from build123d import *

# Parameters (mm, degrees)
F1_DEPTH = 10
F2_T     = -1
F3_R     = 10.6640979673
F4_DEPTH = 25


with BuildPart() as f1:
    # F0 (on Top) → F1 (new body)
    with BuildSketch(Plane.XY):
        Polygon((-31.0254581273, 32.8216664493), (-59.7648322582, 20.7380689681), (-49.9673187733, 12.5734750181), (-42.7824743092, 8.6544696242), (-40.7788045704, 6.7279691546), (-40.7788045704, 2.8554322198), (-41.5555574, -1.3681541895), (-41.5555574, -3.4556735773), (-38.4888425469, -7.9726679251), (-31.0126114637, -14.5143707892), (-28.6823585629, -19.8181271553), (-26.0819279657, -26.5176091343), (-25.6298921539, -27.6821877156), (-16.0601455718, -22.7309465408), (-4.7972491011, -17.4878742546), (0, -16.4924804121), (12.7747104677, -16.4924804121), (15.1070067659, -18.5332398809), (16.0779468715, -21.3716309518), (16.0779468715, -23.5076975077), (15.1070067659, -26.5176091343), (18.6152737588, -32.1685001254), (18.6152737588, -43.598935008), (23.5140342265, -51.1103607714), (25.8403085172, -50.369720906), (28.2073356211, -49.6192015707), (31.2671549618, -48.984143883), (32.1908704937, -47.136709094), (32.7681936324, -45.3470014036), (34.5001667738, -44.6542128921), (35.8280129731, -42.9799742997), (36.2321399152, -40.0933548808), (35.2506898344, -37.0335392654), (33.0568552017, -33.1654660404), (30.863026157, -30.2788466215), (28.0862059444, -27.9229115695), (27.8792269528, -24.5023760945), (27.8792269528, -21.8466855586), (26.8400404602, -20.3456450254), (23.7224902958, -18.7291372567), (22.8264033794, -14.0075832605), (22.8264033794, 0), (33.3115458488, 5.0620483235), (45.0685583055, 10.6139723212), (46.1755990982, 11.7365671322), (45.0685583055, 13.5532263666), (27.7596209198, 22.3709885031), (6.5316753462, 32.8216664493), (-10.4506798089, 40.6596809626), align=None)
    extrude(amount=F1_DEPTH)

    # F2
    f2_openings = [f1.faces().sort_by_distance(p)[0] for p in [
        (-4.783125, 4.353197, 10),
    ]]
    offset(amount=F2_T, openings=f2_openings, kind=Kind.INTERSECTION)

    # F3 (on face) → F4 (cut)
    with BuildSketch(Plane.XY.offset(1)):
        with Locations((-9.2489561066, 8.1327119842)):
            Circle(F3_R)
    extrude(amount=-F4_DEPTH, mode=Mode.SUBTRACT)


solid = f1.part
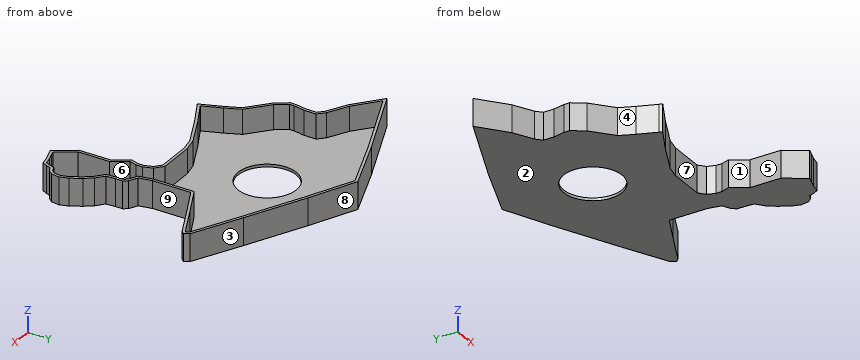
Read the model definition and answer for the solid it produces. Units are mm, in the model's axes. Face numbers are marked on the shaded views. A direction names the side the tool comes from. Coordinates: 2 decimals unless noted, no trailing zeros. Loops run counter-clockwise (first coordinate to the right, second up) from the corner with the lowest first, then second, coordinate; pieces in that order, holes last.
Q1. Consider probe 1 along Y at (x, z) = (24, 6.5); probe 2 along X at (y, z) = (-25, 2); probe 3 along Z at (x, y) = (-43, 25). Determine where each line is inside the solid, lowest interval first.
Q2. The part is cut by section C-C on x = 11. Write down the section's boundary in (y, z), and give its area (3 significant figures).
Q3. The part is cut by section A-A on x = -7. Write down the section's boundary in (y, z).
Q4. Each of these flat-tipped pins is pushed along its axis until it touches: pin 1 Ø1.9 at (y, z) = (-23, 6) entering from -X; pin 2 Ø1.5 at (x, z) = (5, 7.5) entering from -Y; pin 3 Ø3 at (y, z) = (-8, 4) entering from +X. Where does it stop, or does it pass through?
Q5. The mould has two halves that part along X. Classify the marked faces 1, 2, 3 and 4: +X half, -X half, draft (parallel to the pull), parting line (faces both ways), or undercut.
Q6. Which of the six approach directions +Z, -Z, +X, -X, +Y, -Y give full straight-line access (tool end or side, diameter ignored) to the marked faces 5, 6, 7, 8 and 9?
Q7. The part is cut by section B-B on y = 25.5. Write down the section's boundary in (x, z).
Results below:
1. probe 1: y = -50.96 to -49.91, -20 to -18.87, 0.57 to 1.68, 23.11 to 24.22
1. probe 2: x = -26.67 to -25.6, -22.62 to -20.45, 15.6 to 16.65, 26.91 to 27.91
1. probe 3: z = 0 to 1
2. outline: (-16.49, 0) - (30.62, 0) - (30.62, 10) - (29.51, 10) - (29.51, 1) - (-15.49, 1) - (-15.49, 10) - (-16.49, 10) - close
2. area: 66.1 mm2
3. outline: (-18.51, 0) - (-2.29, 0) - (-2.29, 1) - (-17.41, 1) - (-17.41, 10) - (-18.51, 10) - close; (18.56, 0) - (39.07, 0) - (39.07, 10) - (37.97, 10) - (37.97, 1) - (18.56, 1) - close
4. pin 1: stops at x = -27.82
4. pin 2: stops at y = -16.49
4. pin 3: stops at x = 22.83
5. face 1: undercut
5. face 2: draft
5. face 3: +X half
5. face 4: -X half
6. face 5: +Z, -Z, -X, -Y
6. face 6: +Z
6. face 7: +Z, -Z, -Y
6. face 8: +Z, -Z, +X, +Y
6. face 9: +Z, -Z, +X
7. outline: (-48.44, 0) - (21.4, 0) - (21.4, 10) - (19.14, 10) - (19.14, 1) - (-45.86, 1) - (-45.86, 10) - (-48.44, 10) - close
